For this review, take the finished solid that the model builds, in its own axes (mm). A direction names the side the tool comes from. Give positions to 0.01 mm unless a question says otherwise; leave off trailing zeros. Order: outer loops, then holes, each group sorted by start corner. A loop starts at its lowest first (then second) coordinate and runs counter-clockwise, first axis right, second up.
from build123d import *

# Parameters (mm, degrees)
F0_W     = 66.04
F0_H     = 50.8
F1_DEPTH = 25.4
F2_W     = 40.64
F2_H     = 25.4
F2_W_2   = 25.4
F3_DEPTH = 17.78
F4_W     = 40.64
F4_H     = 43.18
F5_DEPTH = 15.24
F6_W     = 25.4
F6_H     = 25.4
F7_DEPTH = 17.78
F8_W     = 25.4
F8_H     = 66.04
F9_DEPTH = 17.78


with BuildPart() as f1:
    # F0 (on Front) → F1 (new body)
    with BuildSketch(Plane.XZ):
        with Locations((-47.104301, -14.145544)):
            Rectangle(F0_W, F0_H)
    extrude(amount=-F1_DEPTH)

    # F2 (on face) → F3 (join)
    with BuildSketch(Plane.XZ):
        with Locations((-59.804301, -1.445544)):
            Rectangle(F2_W, F2_H)
        with Locations((-59.804301, -26.845544)):
            Rectangle(F2_W, F2_H)
        with Locations((-26.784301, -1.445544)):
            Rectangle(F2_W_2, F2_H)
    extrude(amount=F3_DEPTH)

    # F4 (on face) → F5 (join)
    with BuildSketch(Plane.XY.offset(11.254456)):
        with Locations((-59.804301, 3.81)):
            Rectangle(F4_W, F4_H)
    extrude(amount=F5_DEPTH)

    # F6 (on face) → F7 (cut)
    with BuildSketch(Plane.XZ.offset(17.78)):
        with Locations((-26.784301, -1.445544)):
            Rectangle(F6_W, F6_H)
    extrude(amount=-F7_DEPTH, mode=Mode.SUBTRACT)

    # F8 (on face) → F9 (join)
    with BuildSketch(Plane(origin=(-80.124301, 0, 0), x_dir=(0, -1, 0), z_dir=(-1, 0, 0))):
        with Locations((5.08, -6.525544)):
            Rectangle(F8_W, F8_H)
    extrude(amount=F9_DEPTH)


solid = f1.part
1) Clearance check with flat-ended pins moving along their axes: pin 1 (7.5 mm diameter, centred on x = -21.5, y = 18, fed in from +Z); pin 2 (9 mm diameter, centred on y = 20.5, z = 0, fed in from -X); pin 3 (10 mm diameter, centred on x = -36, z = 3, fed in from -Y); pin 4 (19.5 mm diameter, centred on x = -93, z = 2.5, fed in from +Y). State where each tip first meets the part, or that it passes through.
Answer sheet:
pin 1: stops at z = 11.25
pin 2: stops at x = -80.12
pin 3: stops at y = -17.78
pin 4: stops at y = 7.62
2) We need section D-D on z = 13. Give the boundary of the cut face in (x, y), then the cut area to 3 significant figures.
Answer sheet:
outline: (-97.9, -17.78) - (-39.48, -17.78) - (-39.48, 25.4) - (-80.12, 25.4) - (-80.12, 7.62) - (-97.9, 7.62) - close
area: 2,210 mm2
3) We need section B-B on y = 16. Give the boundary of the cut face in (x, z).
Answer sheet:
outline: (-80.12, -39.55) - (-14.08, -39.55) - (-14.08, 11.25) - (-39.48, 11.25) - (-39.48, 26.49) - (-80.12, 26.49) - close
4) We need section C-C on x = -86. Give the boundary of the cut face in (y, z).
Answer sheet:
outline: (-17.78, -39.55) - (7.62, -39.55) - (7.62, 26.49) - (-17.78, 26.49) - close
5) We need section A-A on z = -18. Give the boundary of the cut face in (x, y), then the cut area to 3 significant figures.
Answer sheet:
outline: (-97.9, -17.78) - (-39.48, -17.78) - (-39.48, 0) - (-14.08, 0) - (-14.08, 25.4) - (-80.12, 25.4) - (-80.12, 7.62) - (-97.9, 7.62) - close
area: 2,850 mm2
6) To check wall thickness, follow line 1 (Y direction, x = -35, z = -18); line 2 (Y direction, x = -84, z = 10); line 3 (X direction, y = 13, z = 12). State the ranges of each line that lie inside material, in increasing order.
Answer sheet:
line 1: y = 0 to 25.4
line 2: y = -17.78 to 7.62
line 3: x = -80.12 to -39.48
7) Tool access review of faces 1 (the face through (-80.124, 16, -7)), 2 (the face through (-68, -17.78, -7)), 3 (the face through (-97.904, -5, -6)), 4 (the face through (-27, 13, 11.254)), 5 (the face through (-27, 0, -14)): name each direction out of +Z, -Z, +X, -X, +Y, -Y from which nothing blocks a thin tool from reaching the whole face with its end or side.
Answer sheet:
face 1: +Z, -Z, -X, +Y
face 2: +Z, -Z, +X, -X, -Y
face 3: +Z, -Z, -X, +Y, -Y
face 4: +Z, +X, +Y, -Y
face 5: +Z, -Z, +X, -Y
